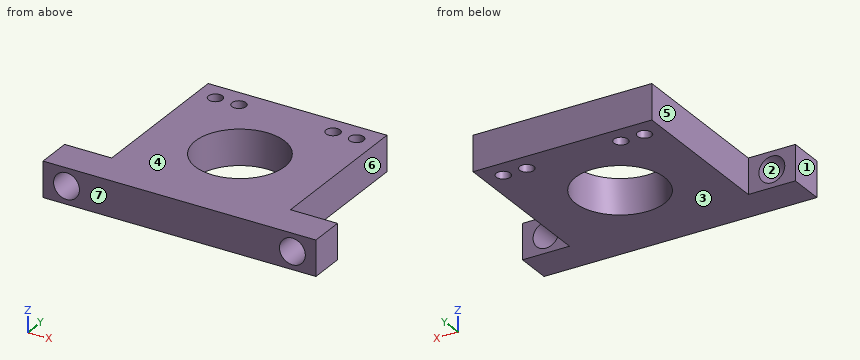
```python
from build123d import *

# Parameters (mm, degrees)
SKETCH1_R           = 9.5
BOSS_EXTRUDE1_DEPTH = 7.5
SKETCH2_R           = 1.5
CUT_EXTRUDE2_DEPTH  = 51.776470929
SKETCH3_R           = 2.75
CUT_EXTRUDE3_DEPTH  = 45.938847337


with BuildPart() as part:
    # Sketch1 → Boss-Extrude1 (new body)
    with BuildSketch(Plane.XY):
        Polygon((-29, 0), (29, 0), (29, 7.5), (19, 7.5), (19, 41), (-19, 41), (-19, 7.5), (-29, 7.5), align=None)
        with Locations((0, 21)):
            Circle(SKETCH1_R, mode=Mode.SUBTRACT)
    extrude(amount=-BOSS_EXTRUDE1_DEPTH)

    # Sketch2 → Cut-Extrude2 (cut, through all)
    with BuildSketch(Plane.XY):
        with Locations((10, 37)):
            Circle(SKETCH2_R)
        with Locations((15, 37)):
            Circle(SKETCH2_R)
        with Locations(Location((-15, 37, 0), (0, 0, 180))):
            Circle(SKETCH2_R)
        with Locations(Location((-10, 37, 0), (0, 0, 180))):
            Circle(SKETCH2_R)
    extrude(amount=-CUT_EXTRUDE2_DEPTH, mode=Mode.SUBTRACT)

    # Sketch3 → Cut-Extrude3 (cut, through all)
    with BuildSketch(Plane(origin=(0, 7.5, 0), x_dir=(1, 0, 0), z_dir=(0, 1, 0))):
        with Locations(Location((-24, 3.75, 0), (0, 0, 180))):
            Circle(SKETCH3_R)
        with Locations(Location((24, 3.75, 0), (0, 0, 180))):
            Circle(SKETCH3_R)
    extrude(amount=-CUT_EXTRUDE3_DEPTH, mode=Mode.SUBTRACT)


solid = part.part
```
Build history of the part. All positions in model axes, mm. Face numbers are marked on the shaded views. A direction names the side the tool comes from. Round coordinates to 2 decimals unless told otherwise and drop trailing zeros. Write each loop counter-clockwise with the first axis right and the second up, starting at its lowest first coordinate (ties: lowest second). Pieces come first, ordered by that corner, then holes. Notation, with made-up numbers: (-6.75, 25) - (1.25, 25) arc R14 cw to (1.25, 40) - close; hole circle Ø10 at (7, 72). An arc over 180 degrees is marked (long way). Write each question's results on one line, items separated by ' | '. Start each with the question number.
Item 1: Which spindle directions (+Z, -Z, +X, -X, +Y, -Y) get a long thin tool onto all of the face, cutting with end or side? Do the marked faces 5, 6 and 7. Say none if no direction does.
Item 2: Drop flat-ended pins along their axis: P1, Ø4.5, axis at x = -24, z = -3.75, coming from the +Y side; P2, Ø3, axis at y = 17, z = -5, coming from the +X side; P3, Ø2, axis at x = 26, z = -2, coming from the +Y side; P4, Ø2, axis at y = 31.5, z = -2.5, coming from the -X side. Give the stop position or say it passes through.
Item 3: Mould opens along Z. For the marked faces 1, 2, 3 and 4 say: pulls with the +Z half, pulls with the -Z half, needs draft (parallel to the pull), parting line crosses it, or undercut.
Item 4: Saw through at B-B (z = -2.5). Write the cut outline in (x, y).
Item 5: Wall check: L1, parallel to Z at x = -24, y = 2; L2, parallel to Y at x = 15, z = -4.25; L3, parallel to X at y = 3, z = -2. Give the ranges that are in metal, low to high. Write a range as [from, to].
Item 6: Saw through at D-D (y = 13). Write the cut outline in (x, z).
Item 7: Saw through at A-A (x = -24). Write the cut outline in (y, z).
Item 8: Saw through at C-C (y = 37). Write the cut outline in (x, z).
Results are:
1) face 5: +Z, -Z, -X, +Y | face 6: +Z, -Z, +X, +Y | face 7: +Z, -Z, +X, -X, -Y
2) P1: passes through | P2: stops at x = 19 | P3: stops at y = 7.5 | P4: stops at x = -19
3) face 1: needs draft | face 2: undercut | face 3: pulls with the -Z half | face 4: pulls with the +Z half
4) outline: (-29, 0) - (-26.45, 0) - (-26.45, 7.5) - (-29, 7.5) - close; (-21.55, 0) - (21.55, 0) - (21.55, 7.5) - (19, 7.5) - (19, 41) - (-19, 41) - (-19, 7.5) - (-21.55, 7.5) - close; (26.45, 0) - (29, 0) - (29, 7.5) - (26.45, 7.5) - close; hole circle Ø3 at (-15, 37); hole circle Ø3 at (-10, 37); hole circle Ø19 at (0, 21); hole circle Ø3 at (10, 37); hole circle Ø3 at (15, 37)
5) L1: z = [-7.5, -6.5], [-1, 0] | L2: y = [0, 35.5], [38.5, 41] | L3: x = [-29, -26.12], [-21.88, 21.88], [26.12, 29]
6) outline: (-19, -7.5) - (-5.12, -7.5) - (-5.12, 0) - (-19, 0) - close; (5.12, -7.5) - (19, -7.5) - (19, 0) - (5.12, 0) - close
7) outline: (0, -7.5) - (7.5, -7.5) - (7.5, -6.5) - (0, -6.5) - close; (0, -1) - (7.5, -1) - (7.5, 0) - (0, 0) - close
8) outline: (-19, -7.5) - (-16.5, -7.5) - (-16.5, 0) - (-19, 0) - close; (-13.5, -7.5) - (-11.5, -7.5) - (-11.5, 0) - (-13.5, 0) - close; (-8.5, -7.5) - (8.5, -7.5) - (8.5, 0) - (-8.5, 0) - close; (11.5, -7.5) - (13.5, -7.5) - (13.5, 0) - (11.5, 0) - close; (16.5, -7.5) - (19, -7.5) - (19, 0) - (16.5, 0) - close
